Read the model definition and answer for the solid it produces. Units are mm, in the model's axes. A direction names the side the tool comes from. Give positions to 0.01 mm unless a question says otherwise; leave off trailing zeros. Put each result on its own line as item: value.
Autodesk Inventor part; units mm, degrees
ref_plane "YZ Plane" through (0, 0, 0) normal (1, 0, 0) x (0, 1, 0)
ref_plane "XZ Plane" through (0, 0, 0) normal (0, 1, 0) x (-1, 0, 0)
ref_plane "XY Plane" through (0, 0, 0) normal (0, 0, 1) x (1, 0, 0)
sketch "Sketch1" plane through (0, 0, 0) normal (0, 0, 1) x (1, 0, 0)
  line L0 (0.6703, -50.425) -> (0.6703, 149.575)
  line L1 (0.6703, 149.575) -> (-359.3297, 149.575)
  line L2 (-359.3297, 149.575) -> (-359.3297, -50.425)
  line L3 (-359.3297, -50.425) -> (0.6703, -50.425)
  line L4 (0.6703, -50.425) -> (0.6703, 149.575)
  point P0 (0, 0)
  dimension "d67" = 360
extrude "Extrusion1" add sketch "Sketch1" along normal blind 15
sketch "Sketch7" plane through (0, 0, 0) normal (0, 0, -1) x (-1, 0, 0)
  line L0 (-0.6703, 149.575) -> (359.3297, 149.575)
  line L1 (-0.6703, 149.575) -> (359.3297, 149.575)
  line L2 (359.3297, 149.575) -> (359.3297, -50.425)
  line L3 (-0.6703, -50.425) -> (-0.6703, 149.575)
  line L4 (-0.6703, 149.575) -> (-0.6703, 129.575)
  line L5 (-0.6703, 149.575) -> (-0.6703, 119.575)
  line L6 (-0.6703, 119.575) -> (-0.6703, 117.575)
  circle A0 centre (56.8297, 102.575) radius 1.5
  circle A1 centre (56.8297, 117.575) radius 1.5
  circle A2 centre (21.8297, 102.575) radius 1.5
  circle A3 centre (21.8297, 117.575) radius 1.5
  line L7 (359.3297, 149.575) -> (359.3297, -50.425)
  line L8 (-0.6703, 117.575) -> (-0.6703, 119.575)
  line L9 (-0.6703, 117.575) -> (-0.6703, 120.575)
  circle A4 centre (300.6557, 89.6777) radius 1.59
  circle A5 centre (300.6557, 74.6777) radius 1.59
  line L10 (16.8297, 102.575) -> (21.8297, 102.575)
  point P0 (0, 0)
  point P1 (300.6557, 74.6777)
  point P2 (340.6556, 74.6777)
  point P3 (340.6556, 89.6777)
  point P4 (335.6556, 88.0877)
  dimension "d70" = 20
  dimension "d155" = 3
hole "Hole10" at (-56.8297, 102.575, 0) at (-56.8297, 117.575, 0) at (-21.8297, 117.575, 0) at (-21.8297, 102.575, 0) direction (0, 0, 1) diameter 3 end through all
hole "Hole11" at (-300.6557, 74.6777, 0) at (-300.6557, 89.6777, 0) at (-340.6556, 74.6777, 0) at (-340.6556, 89.6777, 0) direction (0, 0, 1) diameter 3 end through all
sketch "Sketch11" plane through (0, 0, 15) normal (0, 0, 1) x (1, 0, 0)
  circle A0 centre (-21.8297, 117.575) radius 1.5
  circle A1 centre (-56.8297, 102.575) radius 1.5
  circle A2 centre (-56.8297, 117.575) radius 1.5
  circle A3 centre (-21.8297, 102.575) radius 1.5
  line L0 (0.6703, -50.425) -> (0.6703, 149.575)
  line L1 (0.6703, 149.575) -> (-359.3297, 149.575)
  line L2 (-359.3297, 149.575) -> (-359.3297, -50.425)
  line L3 (-359.3297, -50.425) -> (0.6703, -50.425)
  circle A4 centre (-56.8297, 102.575) radius 1.5
  circle A5 centre (-340.6556, 74.6777) radius 1.5
  circle A6 centre (-340.6556, 89.6777) radius 1.5
  circle A7 centre (-340.6556, 74.6777) radius 1.5
  circle A8 centre (-300.6557, 74.6777) radius 1.5
  circle A9 centre (-300.6557, 89.6777) radius 1.5
  circle A10 centre (-340.6556, 89.6777) radius 1.5
  circle A11 centre (-21.8297, 117.575) radius 1.5
  circle A12 centre (-56.8297, 102.575) radius 1.5
  circle A13 centre (-56.8297, 117.575) radius 1.5
  circle A14 centre (-21.8297, 102.575) radius 1.5
  line L4 (0.6703, -50.425) -> (0.6703, 149.575)
  line L5 (0.6703, 149.575) -> (-359.3297, 149.575)
  line L6 (-359.3297, 149.575) -> (-359.3297, -50.425)
  line L7 (-359.3297, -50.425) -> (0.6703, -50.425)
  point P0 (0, 0)
hole "Hole12" at (-56.8297, 117.575, 15) at (-56.8297, 102.575, 15) at (-21.8297, 102.575, 15) at (-21.8297, 117.575, 15) at (-300.6557, 74.6777, 15) at (-300.6557, 89.6777, 15) at (-340.6556, 89.6777, 15) at (-340.6556, 74.6777, 15) direction (0, 0, -1) diameter 3 end through all countersink diameter 6 countersink angle 90
sketch "Sketch12" plane through (0, 0, 0) normal (0, 0, -1) x (-1, 0, 0)
  circle A0 centre (294.6557, 123.5777) radius 4
  circle A1 centre (346.6557, 123.5777) radius 4
  point P0 (0, 0)
hole "Hole13" at (-294.6557, 123.5777, 0) at (-346.6557, 123.5777, 0) direction (0, 0, 1) diameter 8 end through all
sketch "Sketch13" plane through (0, 0, 15) normal (0, 0, 1) x (1, 0, 0)
  circle A0 centre (-346.6557, 123.5777) radius 4
  circle A1 centre (-294.6557, 123.5777) radius 4
  point P0 (0, 0)
hole "Hole14" at (-346.6557, 123.5777, 15) at (-294.6557, 123.5777, 15) direction (0, 0, -1) diameter 12 depth 8
properties part number "Base de mdf"
(1) Which of the six approach directions +Z, -Z, +X, -X, +Y, -Y give full straight-line access (tool end or side, diameter ignored) to faces 1 (the face through (-182, -50.425, 7)), 2 (the face through (-290.7, 122.3, 7))?
Result:
face 1: +Z, -Z, +X, -X, -Y
face 2: +Z
(2) Straight lines are drawn through the part: line 1 along X through (y, z) = (122.5, 6.75); line 2 along Y through (x, z) = (-344, 13.5) (3 decimals). For each, find the intervals that lie inside material, in ascending order. Write a range as from..to.
Result:
line 1: x = -359.33..-350.51, -342.8..-298.51, -290.8..0.67
line 2: y = -50.425..118.197, 128.958..149.575
(3) For a pull along X with two mould halves and no side action, classify faces 3 (the face through (-343.005, 128.339, 10.944)), 4 (the face through (-182, 51, 0)), 5 (the face through (0.67, 48, 7)), 6 (the face through (-291.005, 128.339, 10.944)) as +X half, -X half, draft (parallel to the pull), parting line (faces both ways), or undercut.
Result:
face 3: undercut
face 4: draft
face 5: +X half
face 6: undercut
(4) Given pin 1 Ø4 at (x, y) = (-300.66, 89.68) entering from -Z; pin 2 Ø1.8 at (x, y) = (-340.66, 74.68) entering from +Z; pin 3 Ø9.5 at (x, y) = (-294.66, 123.58) entering from +Z; pin 4 Ø5 at (x, y) = (-300.66, 74.68) entering from +Z, each flat-ended and moving along its own axis, determine where each tip first touches the part or whether it passes through.
Result:
pin 1: stops at z = 0
pin 2: passes through
pin 3: stops at z = 7
pin 4: stops at z = 14.5
